CAD build for the part. Positions are in the model's coordinates, mm. A direction names the side the tool comes from. Round coordinates to 2 decimals unless told otherwise and drop trailing zeros. Order: outer loops, then holes, each group sorted by start corner. A loop starts at its lowest first (then second) coordinate and runs counter-clockwise, first axis right, second up. Notation, with made-up numbers: M 1.25,-1.5 L 18.25,-1.5 A28 ccw 18.25,26.5 Z; hole C -10,-32.75 d8. An arc over 180 degrees is marked long. Answer as a JSON object with one key per item and string values. Group by question number.
```python
from build123d import *

# Parameters (mm, degrees)
F0_W     = 120
F0_H     = 100
F0_R     = 2.2
F1_DEPTH = 12
F2_R     = 3.75
F3_DEPTH = 5
F5_DEPTH = 4
F6_W     = 80
F6_H     = 100
F7_DEPTH = 25
F8_W     = 17
F8_H     = 65
F9_DEPTH = 25
F10_F1_R = 5
F10_F2_R = 5
F10_F3_R = 5


with BuildPart() as f1:
    # F0 (on Top) → F1 (new body)
    with BuildSketch(Plane.XY):
        Rectangle(F0_W, F0_H)
        with Locations((-46.6, -46.6)):
            Circle(F0_R, mode=Mode.SUBTRACT)
        with Locations((-30, -30)):
            Circle(F0_R, mode=Mode.SUBTRACT)
        with Locations((46.6, -46.6)):
            Circle(F0_R, mode=Mode.SUBTRACT)
        with Locations((30, -30)):
            Circle(F0_R, mode=Mode.SUBTRACT)
        with Locations((-46.6, 46.6)):
            Circle(F0_R, mode=Mode.SUBTRACT)
        with Locations((-30, 30)):
            Circle(F0_R, mode=Mode.SUBTRACT)
        with Locations((30, 30)):
            Circle(F0_R, mode=Mode.SUBTRACT)
        with Locations((46.6, 46.6)):
            Circle(F0_R, mode=Mode.SUBTRACT)
    extrude(amount=-F1_DEPTH)

    # F2 (on face) → F3 (cut)
    with BuildSketch(Plane.XY):
        with Locations((-30, 30)):
            Circle(F2_R)
        with Locations((30, 30)):
            Circle(F2_R)
        with Locations((30, -30)):
            Circle(F2_R)
        with Locations((-30, -30)):
            Circle(F2_R)
    extrude(amount=-F3_DEPTH, mode=Mode.SUBTRACT)

    # F4 (on face) → F5 (cut)
    with BuildSketch(Plane(origin=(0, 0, -12), x_dir=(1, 0, 0), z_dir=(0, 0, -1))):
        Polygon((-43.9383677783, 43.4813923112), (-42.5683904062, 47.3457372751), (-45.2300226279, 50.4643449639), (-49.2616322217, 49.7186076888), (-50.6316095938, 45.8542627249), (-47.9699773721, 42.7356550361), align=None)
        Polygon((46.3647294593, 42.5067558376), (50.0272181581, 44.3496276538), (50.2624886989, 48.4428718162), (46.8352705407, 50.6932441624), (43.1727818419, 48.8503723462), (42.9375113011, 44.7571281838), align=None)
        Polygon((-42.702877562, -45.3262509262), (-45.754537837, -42.5881184301), (-49.651660275, -43.8618675039), (-50.497122438, -47.8737490738), (-47.445462163, -50.6118815699), (-43.548339725, -49.3381324961), align=None)
        Polygon((50.5258183882, -45.4176506509), (47.5389646216, -42.6089668707), (43.6131462335, -43.7913162197), (42.6741816118, -47.7823493491), (45.6610353784, -50.5910331293), (49.5868537665, -49.4086837803), align=None)
    extrude(amount=-F5_DEPTH, mode=Mode.SUBTRACT)

    # F6 (on face) → F7 (cut)
    with BuildSketch(Plane.XY):
        with Locations((20, 0)):
            Rectangle(F6_W, F6_H)
    extrude(amount=-F7_DEPTH, mode=Mode.SUBTRACT)

    # F8 (on face) → F9 (cut)
    with BuildSketch(Plane.XY):
        with Locations((-51.5, 0)):
            Rectangle(F8_W, F8_H)
    extrude(amount=-F9_DEPTH, mode=Mode.SUBTRACT)

    # F10: fillet of radius 5 on 5 edges, made by hand

    # F10_f1
    f10_f1_edges = [f1.edges().sort_by_distance(p)[0] for p in [
        (-43, 32.5, -6),
        (-43, -32.5, -6),
    ]]
    fillet(f10_f1_edges, radius=F10_F1_R)

    # F10_f2
    f10_f2_edges = [f1.edges().sort_by_distance(p)[0] for p in [
        (-43, 0, -12),
        (-44.4644660941, -31.0355339059, -12),
        (-44.4644660941, 31.0355339059, -12),
    ]]
    fillet(f10_f2_edges, radius=F10_F2_R)

    # F10_f3
    f10_f3_edges = [f1.edges().sort_by_distance(p)[0] for p in [
        (-54, 32.5, 0),
        (-43, 0, 0),
        (-44.4644660941, -31.0355339059, 0),
        (-44.4644660941, 31.0355339059, 0),
    ]]
    fillet(f10_f3_edges, radius=F10_F3_R)


solid = f1.part
```
Item 1: Drill centre lines: line 1 (Y direction, x = -30, z = -3.3); line 2 (Y direction, x = -30, z = -9.5); line 3 (Y direction, x = -46.6, z = -4.5). Where is each one in solid material? Low to high. Write a range as [from, to].
Item 2: 3-axis set-ups, long thin cutter, end or side, ignore diameter. For faces 1 (the face through (-46, -43.1, -10)), 2 (the face through (-54.08, 33.93, -10.5)), 3 (the face through (-53.92, 34, -1.43)), 4 (the face through (-44.43, 31, -6.01)), 5 (the face through (-32.764, -27.466, -2.465)): which of +Z, -Z, +X, -X, +Y, -Y reach the whole face in a straight line?
Item 3: Cut at D-D, the plane z = -9.25. Give the cut face in (x, y).
Item 4: Cut at C-C, the plane y = 46.6. Give the cut face in (x, z).
Item 5: Cut at B-B, the plane z = -2. Give the cut face in (x, y).
Item 6: Flat gauge pins, fed straight in: pin 1 Ø5 at (x, y) = (-46.6, -46.6) entering from -Z; pin 2 Ø5.5 at (x, y) = (-30, -30) entering from +Z; pin 3 Ø1.6 at (y, z) = (13, -5.5) entering from -X. Where does each tip first touch, or does it go through?
Item 7: Cut at A-A, the plane x = -30. Give the cut face in (y, z).
Item 8: Two-plate mould, pull along Y, no slides. Class faces 6 (the face through (-60, -41, -6)), 7 (the face through (-49.94, -47.81, -10.03)): +Y half, -Y half, draft (parallel to the pull), parting line (faces both ways), or undercut.
Response values:
{
 "1": {"line 1": "[-50, -33.75], [-26.25, 26.25], [33.75, 50]", "line 2": "[-50, -32.2], [-27.8, 27.8], [32.2, 50]", "line 3": "[-50, -48.8], [-44.4, -32.33], [32.33, 44.4], [48.8, 50]"},
 "2": {"face 1": "-Z", "face 2": "-Z, -X", "face 3": "+Z, -X", "face 4": "+Z, -Z, -X", "face 5": "+Z"},
 "3": {"outline": "M -60,-50 L -47.74,-50 L -49.26,-49.72 L -50.63,-45.85 L -47.97,-42.74 L -43.94,-43.48 L -42.57,-47.35 L -44.83,-50 L -20,-50 L -20,50 L -45.57,50 L -43.55,49.34 L -42.7,45.33 L -45.75,42.59 L -49.65,43.86 L -50.5,47.87 L -48.13,50 L -60,50 L -60,33.03 L -48,33.03 A5.53 cw -42.47,27.5 L -42.47,-27.5 A5.53 cw -48,-33.03 L -60,-33.03 Z; hole C -30,-30 d4.4; hole C -30,30 d4.4"},
 "4": {"outline": "M -60,-12 L -50.23,-12 L -50.23,-8 L -48.8,-8 L -48.8,0 L -60,0 Z; M -44.4,-8 L -42.97,-8 L -42.97,-12 L -20,-12 L -20,0 L -44.4,0 Z"},
 "5": {"outline": "M -60,-50 L -20,-50 L -20,50 L -60,50 L -60,33.5 L -48,33.5 A6 cw -42,27.5 L -42,-27.5 A6 cw -48,-33.5 L -60,-33.5 Z; hole C -46.6,-46.6 d4.4; hole C -46.6,46.6 d4.4; hole C -30,-30 d7.5; hole C -30,30 d7.5"},
 "6": {"pin 1": "z = -8", "pin 2": "z = -5", "pin 3": "x = -43"},
 "7": {"outline": "M -50,-12 L -32.2,-12 L -32.2,-5 L -33.75,-5 L -33.75,0 L -50,0 Z; M -27.8,-12 L 27.8,-12 L 27.8,-5 L 26.25,-5 L 26.25,0 L -26.25,0 L -26.25,-5 L -27.8,-5 Z; M 32.2,-12 L 50,-12 L 50,0 L 33.75,0 L 33.75,-5 L 32.2,-5 Z"},
 "8": {"face 6": "draft", "face 7": "undercut"}
}
